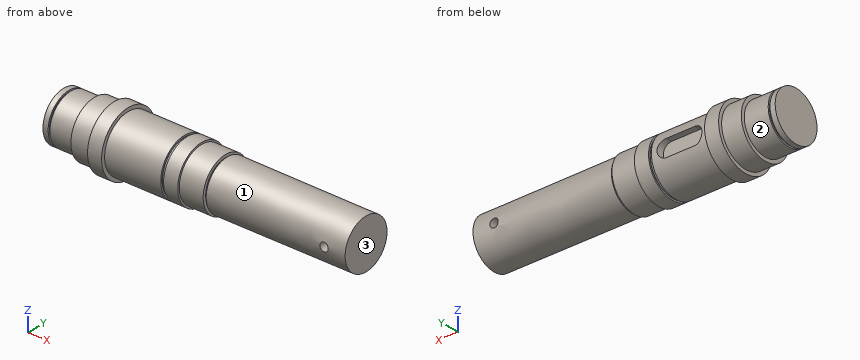
```python
from build123d import *

# Parameters (mm, degrees)
CUT_EXTRUDE1_START = 15
CUT_EXTRUDE1_DEPTH = 6.2
SKETCH3_R          = 3
CUT_EXTRUDE2_DEPTH = 25


with BuildPart() as part:
    # Sketch1 → Revolve1 (revolve)
    with BuildSketch(Plane.XY):
        with BuildLine():
            Line((5.814948309, -5.914886223), (5.814948309, 11.585113777))
            Line((5.814948309, 11.585113777), (9.483069109, 11.585113777))
            Line((9.483069109, 11.585113777), (9.483069109, 10.535113777))
            Line((9.483069109, 10.535113777), (10.783069109, 10.535113777))
            Line((10.783069109, 10.535113777), (10.783069109, 11.585113777))
            Line((10.783069109, 11.585113777), (27.814948309, 11.585113777))
            Line((27.814948309, 11.585113777), (27.814948309, 14.085113777))
            Line((27.814948309, 14.085113777), (41.814948309, 14.085113777))
            Line((41.814948309, 14.085113777), (41.814948309, 16.585113777))
            Line((41.814948309, 16.585113777), (51.814948309, 16.585113777))
            Line((51.814948309, 16.585113777), (51.814948309, 14.085113777))
            Line((51.814948309, 14.085113777), (91.814948309, 14.085113777))
            Line((91.814948309, 14.085113777), (91.814948309, 13.045113777))
            ThreePointArc((91.814948309, 13.045113777), (91.873526953, 12.90369242), (92.014948309, 12.845113777))
            Line((92.014948309, 12.845113777), (93.614948309, 12.845113777))
            ThreePointArc((93.614948309, 12.845113777), (93.756369665, 12.90369242), (93.814948309, 13.045113777))
            Line((93.814948309, 13.045113777), (93.814948309, 14.085113777))
            Line((93.814948309, 14.085113777), (103.914948309, 14.085113777))
            Line((103.914948309, 14.085113777), (103.914948309, 12.835113777))
            Line((103.914948309, 12.835113777), (120.914948309, 12.835113777))
            Line((120.914948309, 12.835113777), (120.914948309, 10.767496152))
            Line((120.914948309, 10.767496152), (122.214948309, 10.767496152))
            Line((122.214948309, 10.767496152), (122.214948309, 11.817496152))
            Line((122.214948309, 11.817496152), (220.914948309, 11.58768633))
            Line((220.914948309, 11.58768633), (220.914948309, -5.914886223))
            Line((220.914948309, -5.914886223), (5.814948309, -5.914886223))
        make_face()
    revolve(axis=Axis((221.999449802, -5.914886223, 0), (-1, 0, 0)))

    # Sketch2 → Cut-Extrude1 (cut)
    with BuildSketch(Plane(origin=(0, 0, 0), x_dir=(1, 0, 0), z_dir=(0, 1, 0)).offset(CUT_EXTRUDE1_START)):
        with BuildLine():
            Line((61.814948309, 6), (81.814948309, 6))
            ThreePointArc((81.814948309, 6), (87.814948309, 0), (81.814948309, -6))
            Line((81.814948309, -6), (61.814948309, -6))
            ThreePointArc((61.814948309, -6), (55.814948309, 0), (61.814948309, 6))
        make_face()
    extrude(amount=-CUT_EXTRUDE1_DEPTH, mode=Mode.SUBTRACT)

    # Sketch3 → Cut-Extrude2 (cut, symmetric)
    with BuildSketch(Plane(origin=(0, 0, 0), x_dir=(1, 0, 0), z_dir=(0, 1, 0))):
        with Locations(Location((205.914948309, 0, 0), (0, 0, 145.09305634))):
            Circle(SKETCH3_R)
    extrude(amount=CUT_EXTRUDE2_DEPTH, both=True, mode=Mode.SUBTRACT)


solid = part.part
```
The listing builds one solid part. Answer for the finished solid, in the listing's coordinates (mm). Face numbers are marked on the shaded views. A direction names the side the tool comes from. Round coordinates to 2 decimals unless told otherwise and drop trailing zeros. Order: outer loops, then holes, each group sorted by start corner. A loop starts at its lowest first (then second) coordinate and runs counter-clockwise, first axis right, second up. Notation, with made-up numbers: (37, -37.5) - (56, -37.5) arc R18 cw to (56, -27.5) - close; hole circle Ø5 at (-2, 1.25). An arc over 180 degrees is marked (long way). Put each result on its own line as item: value. Start each with the question number.
(1) Find section B-B (x = 116). Give the vertices of the cut face in (y, z).
(2) Given P1, Ø1.5, axis at x = 114, y = 6, coming from the +Z side; P2, Ø1.5, axis at y = -20, z = 16.5, coming from the +X side; P3, Ø3, axis at x = 54.5, z = -12.5, coming from the +Y side, each flat-ended and moving along its own axis, determine where each tip first touches the part or whether it passes through.
(3) Find section A-A (x = 24). Give the vertices of the cut face in (y, z).
(4) Straight lines are drawn through the part: probe 1 along X at (y, z) = (-13, 0); probe 2 along X at (y, z) = (-5, -0.5); probe 3 along Z at (x, y) = (87, -6). For each, find the intervals that lie inside material, in ascending order. Write a range as from..to.
(5) For the marked faces 1, 2 and 3, determine the directions among +Z, -Z, +X, -X, +Y, -Y from which every point of the face is accessible in a straight line to the end or side of a thin tool.
Reply:
1. outline: circle Ø37.5 at (-5.91, 0)
2. P1: z = 15.06
2. P2: x = 51.81
2. P3: y = 10.79
3. outline: circle Ø35 at (-5.91, 0)
4. probe 1: 5.81..202.91, 208.91..220.91
4. probe 2: 5.81..202.96, 208.87..220.91
4. probe 3: -20..20
5. face 1: +X
5. face 2: -X
5. face 3: +Z, -Z, +X, +Y, -Y
